from build123d import *

# Parameters (mm, degrees)
SKETCH_W        = 15
SKETCH_H        = 33.5
PAD_DEPTH       = 12
SKETCH001_R     = 1
POCKET_DEPTH    = 12.001
SKETCH002_W     = 24.931972
SKETCH002_H     = 6.15048
SKETCH002_W_2   = 25.150666
SKETCH002_H_2   = 6.153969
POCKET001_DEPTH = 9.5
SKETCH003_W     = 17.12865
SKETCH003_H     = 22.5
POCKET002_DEPTH = 1
SKETCH004_W     = 20.925805
SKETCH004_H     = 24.9
POCKET003_DEPTH = 0.5
SKETCH005_W     = 29.02304
SKETCH005_H     = 9.956954
POCKET004_DEPTH = 15.001
SKETCH006_W     = 24.9
SKETCH006_H     = 4.282043
POCKET005_DEPTH = 14.2
SKETCH007_W     = 15.383407
SKETCH007_H     = 4.5
POCKET006_DEPTH = 2.851
SKETCH008_W     = 33.5
SKETCH008_H     = 4
PAD001_DEPTH    = 2
SKETCH009_W     = 4.5
SKETCH009_H     = 1.85
POCKET007_DEPTH = 2


with BuildPart() as part:
    # Sketch → Pad (new body)
    with BuildSketch(Plane.XZ):
        Rectangle(SKETCH_W, SKETCH_H)
    extrude(amount=PAD_DEPTH)

    # Sketch001 (on Face6 of Pad) → Pocket (cut, through all)
    with BuildSketch(Plane.XZ.offset(12)):
        with Locations((-3.5, 14.375)):
            Circle(SKETCH001_R)
        with Locations((3.5, 14.375)):
            Circle(SKETCH001_R)
        with Locations((-3.5, -14.375)):
            Circle(SKETCH001_R)
        with Locations((3.5, -14.375)):
            Circle(SKETCH001_R)
    extrude(amount=-POCKET_DEPTH, mode=Mode.SUBTRACT)

    # Sketch002 (on Face5 of Pocket) → Pocket001 (cut)
    with BuildSketch(Plane.XZ.offset(12)):
        with Locations((0.203806, 15.07524)):
            Rectangle(SKETCH002_W, SKETCH002_H)
        with Locations((0.641204, -15.0769845)):
            Rectangle(SKETCH002_W_2, SKETCH002_H_2)
    extrude(amount=-POCKET001_DEPTH, mode=Mode.SUBTRACT)

    # Sketch003 (on Face2 of Pocket001) → Pocket002 (cut)
    with BuildSketch(Plane(origin=(0, 0, 0), x_dir=(1, 0, 0), z_dir=(0, 1, 0))):
        with Locations((-3.064325, 0)):
            Rectangle(SKETCH003_W, SKETCH003_H)
    extrude(amount=-POCKET002_DEPTH, mode=Mode.SUBTRACT)

    # Sketch004 (on Face2 of Pocket002) → Pocket003 (cut)
    with BuildSketch(Plane(origin=(0, 0, 0), x_dir=(1, 0, 0), z_dir=(0, 1, 0))):
        with Locations((-3.7629025, 0)):
            Rectangle(SKETCH004_W, SKETCH004_H)
    extrude(amount=-POCKET003_DEPTH, mode=Mode.SUBTRACT)

    # Sketch005 (on Face1 of Pocket003) → Pocket004 (cut, through all)
    with BuildSketch(Plane(origin=(-7.5, 0, 0), x_dir=(0, 0, -1), z_dir=(-1, 0, 0))):
        with Locations((0.508849, 8.978477)):
            Rectangle(SKETCH005_W, SKETCH005_H)
    extrude(amount=-POCKET004_DEPTH, mode=Mode.SUBTRACT)

    # Sketch006 (on Face1 of Pocket004) → Pocket005 (cut)
    with BuildSketch(Plane(origin=(-7.5, 0, 0), x_dir=(0, 0, -1), z_dir=(-1, 0, 0))):
        with Locations((0, -0.9910215)):
            Rectangle(SKETCH006_W, SKETCH006_H)
    extrude(amount=-POCKET005_DEPTH, mode=Mode.SUBTRACT)

    # Sketch007 (on Face5 of Pocket005) → Pocket006 (cut, through all)
    with BuildSketch(Plane(origin=(0, -1.15, 0), x_dir=(1, 0, 0), z_dir=(0, 1, 0))):
        with Locations((-1.6917035, 8.75)):
            Rectangle(SKETCH007_W, SKETCH007_H)
        with Locations((-1.6917035, 0)):
            Rectangle(SKETCH007_W, SKETCH007_H)
        with Locations((-1.6917035, -8.75)):
            Rectangle(SKETCH007_W, SKETCH007_H)
    extrude(amount=-POCKET006_DEPTH, mode=Mode.SUBTRACT)

    # Sketch008 (on Face13 of Pocket006) → Pad001 (join)
    with BuildSketch(Plane(origin=(-7.5, 0, 0), x_dir=(0, 0, -1), z_dir=(-1, 0, 0))):
        with Locations((0, 2)):
            Rectangle(SKETCH008_W, SKETCH008_H)
    extrude(amount=PAD001_DEPTH)

    # Sketch009 (on Face16 of Pad001) → Pocket007 (cut)
    with BuildSketch(Plane(origin=(-9.5, 0, 0), x_dir=(0, 0, -1), z_dir=(-1, 0, 0))):
        with Locations((-8.75, 2.075)):
            Rectangle(SKETCH009_W, SKETCH009_H)
        with Locations((0, 2.075)):
            Rectangle(SKETCH009_W, SKETCH009_H)
        with Locations((8.75, 2.075)):
            Rectangle(SKETCH009_W, SKETCH009_H)
    extrude(amount=-POCKET007_DEPTH, mode=Mode.SUBTRACT)


solid = part.part
Can you work these out from the model? Positions are in its coordinate system, mm. A direction names the side the tool comes from. Give positions to 0.01 mm unless a question says otherwise; leave off trailing zeros. Loops run counter-clockwise (first coordinate to the right, second up) from the corner with the lowest first, then second, coordinate; pieces in that order, holes last. Notation, with made-up numbers: (57, 70.25) - (61, 70.25) arc R22 cw to (61, 91.25) - close; hole circle Ø4 at (49, 66.25). An arc over 180 degrees is marked (long way). One line per item, written item: value.
(1) On a 3-axis mill with a long thin cutter (end or side, diameter ignored), from which of +Z, -Z, +X, -X, +Y, -Y can I reach the whole of each face in a straight line? I mean faces 1 (the face through (0, -3, -12)), 2 (the face through (-9, -1.15, 0)), 3 (the face through (-0.5, -0.6, 12.45)), 4 (the face through (0, -2.5, 14)). Say none if no direction works.
Verdict:
face 1: -Z, +X, -Y
face 2: -X
face 3: +Y
face 4: +Z, +X, -Y
(2) If we section it at C-C, the plane x = -3.5: State how many separate pieces and enclosed holes the cut face has, plus the area to 3 significant figures.
Verdict:
separate pieces: 6
enclosed holes: 0
area: 42.6 mm^2
(3) If we mould it in two halves opening along X, with no side actions, what happens to faces 5 (the face through (-3.72, -1.27, 13.4)), 6 (the face through (-2, -3, -6.5)), 7 (the face through (-9, -3, 9))? For each: released by +X, released by -X, zero draft, split by the parting line, or undercut.
Verdict:
face 5: undercut
face 6: undercut
face 7: zero draft
(4) If we section it at D-D, the plane z = -4: List the corners of the cut face in (x, y) for me, plus the area to 3 significant figures.
Verdict:
outline: (-9.5, -4) - (7.5, -4) - (7.5, 0) - (6.7, 0) - (6.7, -1.15) - (-7.5, -1.15) - (-7.5, 0) - (-9.5, 0) - close
area: 51.7 mm^2
(5) If we section it at A-A, the plane x = -1.75: List the corners of the cut face in (y, z) for me.
Verdict:
outline: (-4, -12) - (-2.5, -12) - (-2.5, -16.75) - (0, -16.75) - (0, -12.45) - (-1.15, -12.45) - (-1.15, -11) - (-4, -11) - close; (-4, -6.5) - (-1.15, -6.5) - (-1.15, -2.25) - (-4, -2.25) - close; (-4, 2.25) - (-1.15, 2.25) - (-1.15, 6.5) - (-4, 6.5) - close; (-4, 11) - (-1.15, 11) - (-1.15, 12.45) - (0, 12.45) - (0, 16.75) - (-2.5, 16.75) - (-2.5, 12) - (-4, 12) - close
(6) If we section it at B-B, the plane z = 9: List the corners of the cut face in (x, y) for me, plus the area to 4 significant figures.
Verdict:
outline: (-9.5, -4) - (-7.5, -4) - (-7.5, -3) - (-9.5, -3) - close; (-9.5, -1.15) - (-7.5, -1.15) - (-7.5, 0) - (-9.5, 0) - close; (6, -4) - (7.5, -4) - (7.5, 0) - (6.7, 0) - (6.7, -1.15) - (6, -1.15) - close
area: 9.495 mm^2
(7) I'm going to push flat-ended pins straight in: pin 1 (0.9 mm diameter, centred on x = 1, y = -3, fed in from -Z); pin 2 (4 mm diameter, centred on x = -4, z = -3.5, fed in from +Y); pin 3 (1.6 mm diameter, centred on x = 3.5, z = -14.375, fed in from +Y); pin 4 (1.6 mm diameter, centred on x = -3.5, y = -3.5, fed in from +Z). Where does each tip first touch, or does it pass through?
Verdict:
pin 1: z = -12
pin 2: y = -1.15
pin 3: through
pin 4: z = 12
(8) I need wall thicknesses on line 1 along Z through (x, y) = (-0.5, -3.45); line 2 along Z through (x, y) = (-3.5, -1.7) (3 decimals); line 3 along Z through (x, y) = (3.5, -0.8) (3 decimals). Which ranges of each line are inside material? Lowest first, please.
Verdict:
line 1: -12 to -11, -6.5 to -2.25, 2.25 to 6.5, 11 to 12
line 2: -16.75 to -15.375, -13.375 to -11, -6.5 to -2.25, 2.25 to 6.5, 11 to 13.375, 15.375 to 16.75
line 3: -16.75 to -15.375, -13.375 to -12.45, 12.45 to 13.375, 15.375 to 16.75
